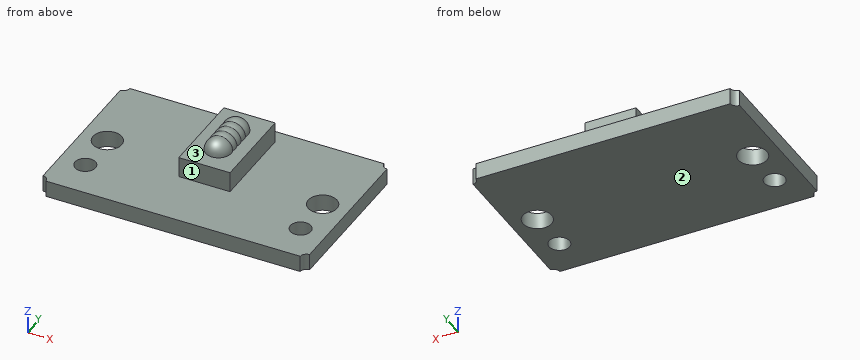
from build123d import *

# Parameters (mm, degrees)
SKETCH1_W           = 26
SKETCH1_H           = 15.8
BOSS_EXTRUDE1_DEPTH = 1.61
SKETCH2_R           = 0.6
CUT_EXTRUDE1_DEPTH  = 1.61
SKETCH3_R           = 1.4
SKETCH3_R_2         = 1
CUT_EXTRUDE2_DEPTH  = 11.61
SKETCH4_W           = 5
SKETCH4_H           = 8.5
BOSS_EXTRUDE2_DEPTH = 2
LPATTERN1_COUNT     = 3
LPATTERN1_PITCH     = 0.8
LPATTERN1_COL_COUNT = 3
LPATTERN1_COL_PITCH = 0.8


with BuildPart() as part:
    # Sketch1 → Boss-Extrude1 (new body)
    with BuildSketch(Plane.XY):
        Rectangle(SKETCH1_W, SKETCH1_H)
    extrude(amount=BOSS_EXTRUDE1_DEPTH)

    # Sketch2 → Cut-Extrude1 (cut)
    with BuildSketch(Plane.XY.offset(1.61)):
        with Locations((-13, 7.9)):
            Circle(SKETCH2_R)
        with Locations((-13, -7.9)):
            Circle(SKETCH2_R)
        with Locations((13, -7.9)):
            Circle(SKETCH2_R)
        with Locations((13, 7.9)):
            Circle(SKETCH2_R)
    extrude(amount=-CUT_EXTRUDE1_DEPTH, mode=Mode.SUBTRACT)

    # Sketch3 → Cut-Extrude2 (cut)
    with BuildSketch(Plane.XY.offset(1.61)):
        with Locations((-10.5, 0)):
            Circle(SKETCH3_R)
        with Locations((10.5, 0)):
            Circle(SKETCH3_R)
        with Locations((-10.5, -4.15)):
            Circle(SKETCH3_R_2)
        with Locations((10.5, -4.15)):
            Circle(SKETCH3_R_2)
    extrude(amount=-CUT_EXTRUDE2_DEPTH, mode=Mode.SUBTRACT)

    # Sketch4 → Boss-Extrude2 (add)
    with BuildSketch(Plane.XY.offset(1.61)):
        with Locations((0, 2.25)):
            Rectangle(SKETCH4_W, SKETCH4_H)
    extrude(amount=BOSS_EXTRUDE2_DEPTH)

    # Sketch5 → Revolve1 (revolve)
    with BuildSketch(Plane.XY.offset(3.61)):
        with BuildLine():
            Line((1.25, 2.25), (-1.25, 2.25))
            ThreePointArc((-1.25, 2.25), (0, 3.5), (1.25, 2.25))
        make_face()
    revolve1 = revolve(axis=Axis((1.25, 2.25, 3.61), (-1, 0, 0)))

    # LPattern1: Revolve1 ×3
    with Locations(*[(0, -i * LPATTERN1_PITCH, 0) for i in range(1, LPATTERN1_COUNT)]):
        add(revolve1)

    # LPattern1 col: Revolve1 ×3
    with Locations(*[(0, i * LPATTERN1_COL_PITCH, 0) for i in range(1, LPATTERN1_COL_COUNT)]):
        add(revolve1)


solid = part.part
Read the model definition and answer for the solid it produces. Units are mm, in the model's axes. Face numbers are marked on the shaded views. A direction names the side the tool comes from. Coordinates: 2 decimals unless noted, no trailing zeros. Order: outer loops, then holes, each group sorted by start corner. A loop starts at its lowest first (then second) coordinate and runs counter-clockwise, first axis right, second up. Notation, with made-up numbers: (61.25, 89) - (112.25, 89) arc R20 cw to (112.25, 120) - close; hole circle Ø9 at (5, 35.25). An arc over 180 degrees is marked (long way). Use one line per item in the form item = value.
(1) Section B-B, the plane y = -4.15 is taken. Give the vertices of the cut face in (x, z).
Computed values:
outline = (-13, 0) - (-11.5, 0) - (-11.5, 1.61) - (-13, 1.61) - close; (-9.5, 0) - (9.5, 0) - (9.5, 1.61) - (-9.5, 1.61) - close; (11.5, 0) - (13, 0) - (13, 1.61) - (11.5, 1.61) - close
(2) Given pin 1 Ø1 at (x, z) = (-5, 2) entering from -Y; pin 2 Ø1.6 at (y, z) = (1, 3) entering from +X; pin 3 Ø4.5 at (x, y) = (-2.5, -3.5) entering from +Z; pin 4 Ø0.6 at (x, z) = (1, 2.5) entering from -Y, each flat-ended and moving along its own axis, determine where each tip first touches the part or whether it passes through.
Computed values:
pin_1 = -7.9
pin_2 = 2.5
pin_3 = 3.61
pin_4 = -2
(3) Which of the six approach directions +Z, -Z, +X, -X, +Y, -Y give full straight-line access (tool end or side, diameter ignored) to the marked faces 1, 2 and 3?
Computed values:
face_1 = +Z, +X, -X, -Y
face_2 = -Z, +X, -X, +Y, -Y
face_3 = +Z
(4) Section A-A, the plane x = 10.5 is taken. Give the vertices of the cut face in (y, z), then the cut area to 3 significant figures.
Computed values:
outline = (-7.9, 0) - (-5.15, 0) - (-5.15, 1.61) - (-7.9, 1.61) - close; (-3.15, 0) - (-1.4, 0) - (-1.4, 1.61) - (-3.15, 1.61) - close; (1.4, 0) - (7.9, 0) - (7.9, 1.61) - (1.4, 1.61) - close
area = 17.7 mm²
(5) Section C-C, the plane z = 0.65 is taken. Give the vertices of the cut face in (x, y), then the cut area to 3 significant figures.
Computed values:
outline = (-13, -7.3) arc R0.6 cw to (-12.4, -7.9) - (12.4, -7.9) arc R0.6 cw to (13, -7.3) - (13, 7.3) arc R0.6 cw to (12.4, 7.9) - (-12.4, 7.9) arc R0.6 cw to (-13, 7.3) - close; hole circle Ø2.8 at (-10.5, 0); hole circle Ø2 at (-10.5, -4.15); hole circle Ø2.8 at (10.5, 0); hole circle Ø2 at (10.5, -4.15)
area = 391 mm²
(6) Straight lines are drawn through the part: L1, parallel to Y at x = -10.5, z = 0.95; L2, parallel to Z at x = 4, y = 2.25; L3, parallel to Y at x = 1.75, z = 1.8. For each, find the intervals that lie inside material, in ascending order.
Computed values:
L1 = -7.9 to -5.15, -3.15 to -1.4, 1.4 to 7.9
L2 = 0 to 1.61
L3 = -2 to 6.5
(7) Section D-D, the plane x = 2 is taken. Give the vertices of the cut face in (y, z).
Computed values:
outline = (-7.9, 0) - (7.9, 0) - (7.9, 1.61) - (6.5, 1.61) - (6.5, 3.61) - (-2, 3.61) - (-2, 1.61) - (-7.9, 1.61) - close
